```python
from build123d import *

# Parameters (mm, degrees)
F0_W     = 76.2
F0_H     = 76.2
F1_DEPTH = 25.4
F3_D     = 6.5278
F3_DEPTH = 16.9333333333
F3_TIP   = 1.9611489744


with BuildPart() as f1:
    # F0 (on Front) → F1 (new body)
    with BuildSketch(Plane.XZ):
        Rectangle(F0_W, F0_H)
    extrude(amount=F1_DEPTH)

    # F3
    with Locations(Plane.XZ.offset(25.4)):
        with Locations((-23.415625, 23.415625), (23.415625, 23.415625), (23.415625, -23.415625), (-23.415625, -23.415625)):
            Hole(F3_D / 2, depth=F3_DEPTH)
            with Locations((0, 0, -(F3_DEPTH + F3_TIP / 2))):  # 118° drill point
                Cone(0, F3_D / 2, F3_TIP, mode=Mode.SUBTRACT)


solid = f1.part
```
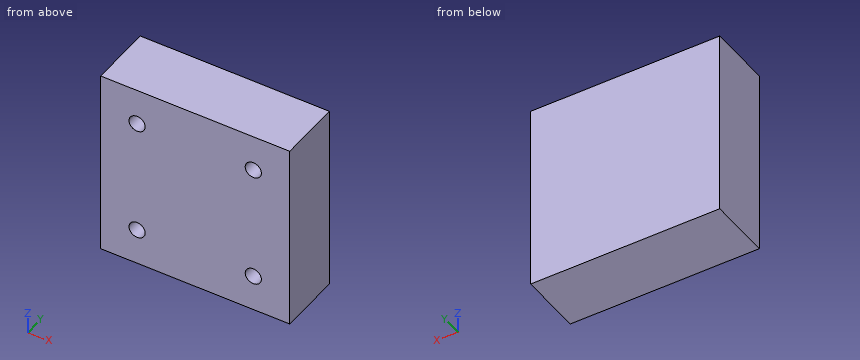
Part model, mm, in its own coordinate system. Round coordinates to 2 decimals unless told otherwise and drop trailing zeros. Order: outer loops, then holes, each group sorted by start corner. A loop starts at its lowest first (then second) coordinate and runs counter-clockwise, first axis right, second up. Notation, with made-up numbers: M 24.5,70 L 70.5,70 A32 cw 70.5,103 Z; hole C 28.25,83 d6. An arc over 180 degrees is marked long. Answer in a Markdown table with one row per item. Add a question column.
Q1. Wall check: L1, parallel to X at y = -10, z = 20.5; L2, parallel to X at y = -13.5, z = 25.5. Give the ranges that are in metal, low to high. Write a range as from..to.
Q2. Cut at A-A on y = -21. Give the cut face in (x, z), and give its area (3 significant figures).
Q3. Pin check, flat tips, straight feed: pin 1 (5 mm diameter, centred on x = -23.42, z = 23.42, fed in from +Y); pin 2 (5 mm diameter, centred on x = 23.42, z = -23.42, fed in from -Y). Stop position of each tip, or through.
Established:
| question | item | result |
|---|---|---|
| 1 | L1 | x = -38.1..-24.88, -21.95..21.95, 24.88..38.1 |
| 1 | L2 | x = -38.1..-25.93, -20.9..20.9, 25.93..38.1 |
| 2 | outline | M -38.1,-38.1 L 38.1,-38.1 L 38.1,38.1 L -38.1,38.1 Z; hole C -23.42,-23.42 d6.53; hole C -23.42,23.42 d6.53; hole C 23.42,-23.42 d6.53; hole C 23.42,23.42 d6.53 |
| 2 | area | 5,670 mm2 |
| 3 | pin 1 | stops at y = 0 |
| 3 | pin 2 | stops at y = -8.01 |
